```python
from build123d import *

# Parameters (mm, degrees)
SKETCH1_W             = 26.5
SKETCH1_H             = 6
BOSS_EXTRUDE1_DEPTH   = 17
SKETCH2_R             = 1.5
CUT_EXTRUDE1_DEPTH    = 1
SKETCH3_R             = 1.3
CUT_EXTRUDE2_DEPTH    = 32.878676259
SKETCH4_R             = 4
CUT_EXTRUDE3_DEPTH    = 33.050741021
SKETCH5_R             = 2.5
CUT_EXTRUDE4_DEPTH    = 1.5
SKETCH6_R             = 1.5
CUT_EXTRUDE8_DEPTH    = 1
SKETCH7_R             = 1.3
CUT_EXTRUDE9_DEPTH    = 32.678068123
CUT_EXTRUDE10_START   = -1
SKETCH8_R             = 2.5
CUT_EXTRUDE10_DEPTH   = 1
CUT_EXTRUDE11_START   = -1
SKETCH9_R             = 1.5
CUT_EXTRUDE11_DEPTH   = 1
SKETCH10_R            = 5.5
SKETCH10_R_2          = 4
BOSS_EXTRUDE2_DEPTH   = 3.5
SKETCH11_R            = 3
SKETCH11_R_2          = 1.3
BOSS_EXTRUDE4_DEPTH   = 2
CUT_EXTRUDE12_START   = -1
SKETCH12_R            = 1.5
CUT_EXTRUDE12_DEPTH   = 1
SKETCH17_W            = 2
SKETCH17_H            = 6
BOSS_EXTRUDE6_DEPTH   = 1.5
SKETCH18_R            = 1
CUT_EXTRUDE17_DEPTH   = 33.050741021
CHAMFER2_SIZE         = 5
CHAMFER2_SIZE2        = 3.5
FILLET11_R            = 3
BOSS_EXTRUDE7_DEPTH   = 2
CUT_EXTRUDE19_DEPTH   = 33.050741021
FILLET13_R            = 5
FILLET14_R            = 3
FILLET15_R            = 3
MIRROR6_OUTLINE_R     = 4
MIRROR6_OUTLINE_R_2   = 2.5
MIRROR6_OUTLINE_R_3   = 1.5
MIRROR6_DEPTH         = 6
MIRROR6_START         = 6
MIRROR6_2_OUTLINE_R   = 4
MIRROR6_2_OUTLINE_R_2 = 1.5
MIRROR6_2_DEPTH       = 2
MIRROR6_START_2       = 8
MIRROR6_3_OUTLINE_R   = 5.5
MIRROR6_3_OUTLINE_R_2 = 4
MIRROR6_3_DEPTH       = 1.5
MIRROR6_START_3       = 1.5
MIRROR6_4_OUTLINE_R   = 1.5
MIRROR6_4_OUTLINE_R_2 = 1.3
MIRROR6_4_OUTLINE_R_3 = 2.5
MIRROR6_4_DEPTH       = 3.5
MIRROR6_START_4       = 1
MIRROR6_5_OUTLINE_R   = 1.5
MIRROR6_5_OUTLINE_R_2 = 1.3
MIRROR6_5_DEPTH       = 6
MIRROR6_START_5       = 2.5
MIRROR6_6_OUTLINE_R   = 1.5
MIRROR6_6_OUTLINE_R_2 = 1.3
MIRROR6_6_DEPTH       = 1.5
CUT_EXTRUDE20_DEPTH   = 34.963215396


# Read off the part's stored shape, not the designer's step: Mirror6
with BuildPart() as part:
    # Sketch1 → Boss-Extrude1 (new body)
    with BuildSketch(Plane(origin=(0, 0, 0), x_dir=(1, 0, 0), z_dir=(0, 1, 0))):
        with Locations((13.25, 3)):
            Rectangle(SKETCH1_W, SKETCH1_H)
    extrude(amount=BOSS_EXTRUDE1_DEPTH)

    # Sketch2 → Cut-Extrude1 (cut)
    with BuildSketch(Plane.XY):
        with Locations((12.5, 5.5)):
            Circle(SKETCH2_R)
    extrude(amount=-CUT_EXTRUDE1_DEPTH, mode=Mode.SUBTRACT)

    # Sketch3 → Cut-Extrude2 (cut, through all)
    with BuildSketch(Plane.XY.offset(-1)):
        with Locations((12.5, 5.5)):
            Circle(SKETCH3_R)
    extrude(amount=-CUT_EXTRUDE2_DEPTH, mode=Mode.SUBTRACT)

    # Sketch4 → Cut-Extrude3 (cut, through all)
    with BuildSketch(Plane.XY):
        with Locations((19.208203932, 11.5)):
            Circle(SKETCH4_R)
    extrude(amount=-CUT_EXTRUDE3_DEPTH, mode=Mode.SUBTRACT)

    # Sketch5 → Cut-Extrude4 (cut)
    with BuildSketch(Plane.XY):
        with Locations((3.5, 5.5)):
            Circle(SKETCH5_R)
    extrude(amount=-CUT_EXTRUDE4_DEPTH, mode=Mode.SUBTRACT)

    # Sketch6 → Cut-Extrude8 (cut)
    with BuildSketch(Plane.XY.offset(-1.5)):
        with Locations((3.5, 5.5)):
            Circle(SKETCH6_R)
    extrude(amount=-CUT_EXTRUDE8_DEPTH, mode=Mode.SUBTRACT)

    # Sketch7 → Cut-Extrude9 (cut, through all)
    with BuildSketch(Plane.XY.offset(-2.5)):
        with Locations((3.5, 5.5)):
            Circle(SKETCH7_R)
    extrude(amount=-CUT_EXTRUDE9_DEPTH, mode=Mode.SUBTRACT)

    # Sketch8 → Cut-Extrude10 (cut)
    with BuildSketch(Plane(origin=(0, 0, -6), x_dir=(-1, 0, 0), z_dir=(0, 0, -1)).offset(CUT_EXTRUDE10_START)):
        with Locations(Location((-3.5, 5.5, 0), (0, 0, 180))):
            Circle(SKETCH8_R)
    extrude(amount=CUT_EXTRUDE10_DEPTH, mode=Mode.SUBTRACT)

    # Sketch9 → Cut-Extrude11 (cut)
    with BuildSketch(Plane(origin=(0, 0, -5), x_dir=(-1, 0, 0), z_dir=(0, 0, -1)).offset(CUT_EXTRUDE11_START)):
        with Locations(Location((-3.5, 5.5, 0), (0, 0, 180))):
            Circle(SKETCH9_R)
    extrude(amount=CUT_EXTRUDE11_DEPTH, mode=Mode.SUBTRACT)

    # Sketch10 → Boss-Extrude2 (add)
    with BuildSketch(Plane(origin=(0, 0, -6), x_dir=(-1, 0, 0), z_dir=(0, 0, -1))):
        with Locations(Location((-19.208203932, 11.5, 0), (0, 0, 90))):
            Circle(SKETCH10_R)
        with Locations(Location((-19.208203932, 11.5, 0), (0, 0, 180))):
            Circle(SKETCH10_R_2, mode=Mode.SUBTRACT)
    extrude(amount=BOSS_EXTRUDE2_DEPTH)

    # Sketch11 → Boss-Extrude4 (add)
    with BuildSketch(Plane(origin=(0, 0, -6), x_dir=(-1, 0, 0), z_dir=(0, 0, -1))):
        with Locations(Location((-12.5, 5.5, 0), (0, 0, 180))):
            Circle(SKETCH11_R)
        with Locations(Location((-12.5, 5.5, 0), (0, 0, 180))):
            Circle(SKETCH11_R_2, mode=Mode.SUBTRACT)
    extrude(amount=BOSS_EXTRUDE4_DEPTH)

    # Sketch12 → Cut-Extrude12 (cut)
    with BuildSketch(Plane(origin=(0, 0, -8), x_dir=(-1, 0, 0), z_dir=(0, 0, -1)).offset(CUT_EXTRUDE12_START)):
        with Locations(Location((-12.5, 5.5, 0), (0, 0, 180))):
            Circle(SKETCH12_R)
    extrude(amount=CUT_EXTRUDE12_DEPTH, mode=Mode.SUBTRACT)

    # Sketch17 → Boss-Extrude6 (add)
    with BuildSketch(Plane.XZ):
        with Locations((6, -3)):
            Rectangle(SKETCH17_W, SKETCH17_H)
        with Locations((20.5, -3)):
            Rectangle(SKETCH17_W, SKETCH17_H)
    extrude(amount=BOSS_EXTRUDE6_DEPTH)

    # Sketch18 → Cut-Extrude17 (cut, through all)
    with BuildSketch(Plane(origin=(0, 0, -6), x_dir=(-1, 0, 0), z_dir=(0, 0, -1))):
        with Locations((-22.5, 0)):
            Circle(SKETCH18_R)
        with Locations((-18.5, 0)):
            Circle(SKETCH18_R)
        with Locations((-8, 0)):
            Circle(SKETCH18_R)
        with Locations((-4, 0)):
            Circle(SKETCH18_R)
    extrude(amount=-CUT_EXTRUDE17_DEPTH, mode=Mode.SUBTRACT)

    # Chamfer2
    chamfer2_edges = [part.edges().sort_by_distance(p)[0] for p in [
        (26.5, 17, -3),
    ]]
    chamfer2_side = [part.faces().sort_by_distance(p)[0] for p in [
        (26.5, 8.5, -3),
    ]]
    chamfer(chamfer2_edges, length=CHAMFER2_SIZE, length2=CHAMFER2_SIZE2, reference=chamfer2_side[0])

    # Fillet11
    fillet11_edges = [part.edges().sort_by_distance(p)[0] for p in [
        (23, 17, -3),
        (26.5, 12, -3),
    ]]
    fillet(fillet11_edges, radius=FILLET11_R)

    # Sketch19 → Boss-Extrude7 (add)
    with BuildSketch(Plane(origin=(0, 0, -6), x_dir=(-1, 0, 0), z_dir=(0, 0, -1))):
        with BuildLine():
            Line((-14.547099294, 14.419606745), (-9.957579288, 7.09251277))
            ThreePointArc((-9.957579288, 7.09251277), (-14.736067977, 7.5), (-13.800160725, 2.796376119))
            Line((-13.800160725, 2.796376119), (-21.591831928, 6.543356218))
            ThreePointArc((-21.591831928, 6.543356218), (-15.108745974, 7.833333333), (-14.547099294, 14.419606745))
        make_face()
    extrude(amount=BOSS_EXTRUDE7_DEPTH)

    # Sketch20 → Cut-Extrude19 (cut, through all)
    with BuildSketch(Plane(origin=(0, 0, -6), x_dir=(-1, 0, 0), z_dir=(0, 0, -1))):
        Polygon((0, 17), (-14.011012575, 17), (-9, 9), (0, 9), align=None)
    extrude(amount=-CUT_EXTRUDE19_DEPTH, mode=Mode.SUBTRACT)

    # Fillet13
    fillet13_edges = [part.edges().sort_by_distance(p)[0] for p in [
        (14.011012575, 17, -3),
    ]]
    fillet(fillet13_edges, radius=FILLET13_R)

    # Fillet14
    fillet14_edges = [part.edges().sort_by_distance(p)[0] for p in [
        (9, 9, -3),
    ]]
    fillet(fillet14_edges, radius=FILLET14_R)

    # Fillet15
    fillet15_edges = [part.edges().sort_by_distance(p)[0] for p in [
        (0, 9, -3),
    ]]
    fillet(fillet15_edges, radius=FILLET15_R)

    # Mirror6 outline → Mirror6 (add)
    with BuildSketch(Plane.XY):
        with BuildLine():
            Line((21.438033315, 17), (16.779018718, 17))
            ThreePointArc((16.779018718, 17), (14.357339523, 16.374410803), (12.541650865, 14.65418795))
            Line((12.541650865, 14.65418795), (9.881617026, 10.40748723))
            ThreePointArc((9.881617026, 10.40748723), (8.792203831, 9.375353518), (7.339196314, 9))
            Line((7.339196314, 9), (3, 9))
            ThreePointArc((3, 9), (0.878679656, 8.121320344), (0, 6))
            Line((0, 6), (0, 0))
            Line((0, 0), (3, 0))
            ThreePointArc((3, 0), (4, 1), (5, 0))
            Line((5, 0), (5, -1.5))
            Line((5, -1.5), (7, -1.5))
            Line((7, -1.5), (7, 0))
            ThreePointArc((7, 0), (8, 1), (9, 0))
            Line((9, 0), (17.5, 0))
            ThreePointArc((17.5, 0), (18.5, 1), (19.5, 0))
            Line((19.5, 0), (19.5, -1.5))
            Line((19.5, -1.5), (21.5, -1.5))
            Line((21.5, -1.5), (21.5, 0))
            ThreePointArc((21.5, 0), (22.5, 1), (23.5, 0))
            Line((23.5, 0), (26.5, 0))
            Line((26.5, 0), (26.5, 11.054333308))
            ThreePointArc((26.5, 11.054333308), (26.361213666, 11.956251462), (25.957695762, 12.774720341))
            Line((25.957695762, 12.774720341), (23.895729077, 15.720387033))
            ThreePointArc((23.895729077, 15.720387033), (22.823464458, 16.660936029), (21.438033315, 17))
        make_face()
        with Locations((19.208203932, 11.5)):
            Circle(MIRROR6_OUTLINE_R, mode=Mode.SUBTRACT)
        with Locations((3.5, 5.5)):
            Circle(MIRROR6_OUTLINE_R_2, mode=Mode.SUBTRACT)
        with Locations((12.5, 5.5)):
            Circle(MIRROR6_OUTLINE_R_3, mode=Mode.SUBTRACT)
    extrude(amount=MIRROR6_DEPTH)

    # Mirror6 2 outline → Mirror6 2 (add)
    with BuildSketch(Plane.XY.offset(MIRROR6_START)):
        with BuildLine():
            Line((14.547099293, 14.419606745), (9.957579288, 7.09251277))
            ThreePointArc((9.957579288, 7.09251277), (10.263932023, 3.5), (13.800160725, 2.796376119))
            Line((13.800160725, 2.796376119), (21.591831928, 6.543356218))
            ThreePointArc((21.591831928, 6.543356218), (23.307661891, 15.166666667), (14.547099293, 14.419606745))
        make_face()
        with Locations((19.208203932, 11.5)):
            Circle(MIRROR6_2_OUTLINE_R, mode=Mode.SUBTRACT)
        with Locations((12.5, 5.5)):
            Circle(MIRROR6_2_OUTLINE_R_2, mode=Mode.SUBTRACT)
    extrude(amount=MIRROR6_2_DEPTH)

    # Mirror6 3 outline → Mirror6 3 (add)
    with BuildSketch(Plane.XY.offset(MIRROR6_START_2)):
        with Locations((19.208203932, 11.5)):
            Circle(MIRROR6_3_OUTLINE_R)
        with Locations((19.208203932, 11.5)):
            Circle(MIRROR6_3_OUTLINE_R_2, mode=Mode.SUBTRACT)
    extrude(amount=MIRROR6_3_DEPTH)

    # Mirror6 4 outline → Mirror6 4 (add)
    # profile 1 of 2: a face of its own
    with BuildSketch(Plane.XY.offset(MIRROR6_START_3)):
        with Locations((12.5, 5.5)):
            Circle(MIRROR6_4_OUTLINE_R)
        with Locations((12.5, 5.5)):
            Circle(MIRROR6_4_OUTLINE_R_2, mode=Mode.SUBTRACT)
    # profile 2 of 2: a face of its own
    with BuildSketch(Plane.XY.offset(MIRROR6_START_3)):
        with Locations((3.5, 5.5)):
            Circle(MIRROR6_4_OUTLINE_R_3)
        with Locations((3.5, 5.5)):
            Circle(MIRROR6_4_OUTLINE_R, mode=Mode.SUBTRACT)
    extrude(amount=MIRROR6_4_DEPTH)

    # Mirror6 5 outline → Mirror6 5 (add)
    with BuildSketch(Plane.XY.offset(MIRROR6_START_4)):
        with Locations((12.5, 5.5)):
            Circle(MIRROR6_5_OUTLINE_R)
        with Locations((12.5, 5.5)):
            Circle(MIRROR6_5_OUTLINE_R_2, mode=Mode.SUBTRACT)
    extrude(amount=MIRROR6_5_DEPTH)

    # Mirror6 6 outline → Mirror6 6 (add)
    with BuildSketch(Plane.XY.offset(MIRROR6_START_5)):
        with Locations((3.5, 5.5)):
            Circle(MIRROR6_6_OUTLINE_R)
        with Locations((3.5, 5.5)):
            Circle(MIRROR6_6_OUTLINE_R_2, mode=Mode.SUBTRACT)
    extrude(amount=MIRROR6_6_DEPTH)

    # Sketch24 → Cut-Extrude20 (cut, through all)
    with BuildSketch(Plane(origin=(0, -2, 0), x_dir=(1, 0, 0), z_dir=(0, 1, 0))):
        Polygon((0, 0), (26.5, 0), (26.5, 6), (26.5, 9.5), (24.708203932, 9.5), (13.708203932, 9.5), (0, 9.5), (0, 6), align=None)
    extrude(amount=CUT_EXTRUDE20_DEPTH, mode=Mode.SUBTRACT)


solid = part.part
```
Input: part model. Units: mm. Frame: model coordinates. A direction names the side the tool comes from. Coordinates: 2 decimals unless noted, no trailing zeros. Order: outer loops, then holes, each group sorted by start corner. A loop starts at its lowest first (then second) coordinate and runs counter-clockwise, first axis right, second up. Notation, with made-up numbers: (-9, 13) - (47, 13) arc R11 ccw to (47, 27) - close; hole circle Ø1 at (-34, 71). An arc over 180 degrees is marked (long way). Put each result on its own line as item: value.
1. Cut plane C-C on x = 22.75. Return the cut outline in (y, z), then the cut area to 3 significant figures.
Report:
outline: (0.97, 0) - (9.64, 0) - (9.64, 9.5) - (7.29, 9.5) - (7.29, 6) - (0.97, 6) - close; (13.36, 0) - (16.7, 0) - (16.7, 6) - (15.71, 6) - (15.71, 9.5) - (13.36, 9.5) - close
area: 88.5 mm2
2. Cut plane B-B on y = 9.5. Return the cut outline in (x, z).
Report:
outline: (9, 0) - (15.74, 0) - (15.74, 9.5) - (14.08, 9.5) - (14.08, 8) - (11.47, 8) - (11.47, 6) - (9, 6) - close; (22.67, 0) - (26.5, 0) - (26.5, 6) - (24.33, 6) - (24.33, 9.5) - (22.67, 9.5) - close
3. Contact query for flat-ended pins moving along their axis: pin 1 Ø5 at (x, y) = (23, 3.5) entering from +Z; pin 2 Ø3.5 at (x, y) = (4, 5) entering from -Z; pin 3 Ø6.5 at (x, y) = (19.21, 11.5) entering from +Z; pin 4 Ø3.5 at (x, y) = (12.5, 8) entering from +Z. Output: stop coordinate, or through.
Report:
pin 1: stops at z = 6
pin 2: stops at z = 1.5
pin 3: passes through
pin 4: stops at z = 8
4. Cut plane A-A on z = 2. Return the cut outline in (x, y), then the cut area to 3 significant figures.
Report:
outline: (0, 0) - (3, 0) arc R1 cw to (5, 0) - (5, -1.5) - (7, -1.5) - (7, 0) arc R1 cw to (9, 0) - (17.5, 0) arc R1 cw to (19.5, 0) - (19.5, -1.5) - (21.5, -1.5) - (21.5, 0) arc R1 cw to (23.5, 0) - (26.5, 0) - (26.5, 11.05) arc R3 ccw to (25.96, 12.77) - (23.9, 15.72) arc R3 ccw to (21.44, 17) - (16.78, 17) arc R5 ccw to (12.54, 14.65) - (9.88, 10.41) arc R3 cw to (7.34, 9) - (3, 9) arc R3 ccw to (0, 6) - close; hole circle Ø3 at (3.5, 5.5); hole circle Ø2.6 at (12.5, 5.5); hole circle Ø8 at (19.21, 11.5)
area: 284 mm2
5. Reachability of faces 4 (the face through (5.885, 6.251, 5.493)), 5 (the face through (25, 0, 3)), 6 (the face through (4.886, 4.925, 1.993)) from +Z, -Z, +X, -X, +Y, -Y: full face, straight path, thin tool, end or side. Return the list, or none.
Report:
face 4: +Z
face 5: +Z, -Z, +X, -Y
face 6: -Z
6. Line query: line 1 along X through (y, z) = (6.5, 0.5); line 2 along X through (y, z) = (6, 2); line 3 along Z through (x, y) = (8.5, 4.75). Output: solid intervals per line, ascending.
Report:
line 1: x = 0.04 to 1.21, 5.79 to 11.38, 13.62 to 26.5
line 2: x = 0 to 2.09, 4.91 to 11.3, 13.7 to 26.5
line 3: z = 0 to 6
7. Draft query along X for faces 1 (the face through (8.811, 9.386, 2.958)), 2 (the face through (16, 6, 0)), 3 (the face through (11, 5.57, 0.49)). Return one class per face: pulls with the +X half, pulls with the -X half, needs draft (parallel to the pull), parting line crosses it, or undercut.
Report:
face 1: pulls with the -X half
face 2: needs draft
face 3: undercut
8. Cut plane D-D on z = 7.5. Return the cut outline in (x, y).
Report:
outline: (9.96, 7.09) arc R3 ccw to (13.8, 2.8) - (21.59, 6.54) arc R5.5 ccw (long way) to (14.55, 14.42) - close; hole circle Ø3 at (12.5, 5.5); hole circle Ø8 at (19.21, 11.5)
